```python
from build123d import *

# Parameters (mm, degrees)
SKETCH1_R           = 1
SKETCH1_R_2         = 8.1
SKETCH1_R_3         = 1.5
BOSS_EXTRUDE1_DEPTH = 3
SKETCH2_W           = 8.84
SKETCH2_H           = 1.2
CUT_EXTRUDE1_DEPTH  = 3
FILLET1_R           = 1
FILLET4_R           = 0.6


with BuildPart() as part:
    # Sketch1 → Boss-Extrude1 (new body)
    with BuildSketch(Plane(origin=(0, 0, 0), x_dir=(1, 0, 0), z_dir=(0, 1, 0))):
        Polygon((0, 0), (0, 20.3), (45, 20.3), (45, 0), (45, -3), (32.5, -3), (32.5, -13), (12.5, -13), (12.5, -3), (0, -3), align=None)
        with Locations(Location((1.4, 18.7, 0), (0, 0, 270))):
            Circle(SKETCH1_R, mode=Mode.SUBTRACT)
        with Locations(Location((1.4, 1.6, 0), (0, 0, 90))):
            Circle(SKETCH1_R, mode=Mode.SUBTRACT)
        with Locations(Location((43.6, 1.6, 0), (0, 0, 270))):
            Circle(SKETCH1_R, mode=Mode.SUBTRACT)
        with Locations(Location((43.6, 18.7, 0), (0, 0, 90))):
            Circle(SKETCH1_R, mode=Mode.SUBTRACT)
        with Locations(Location((9.58, 10.32, 0), (0, 0, 270))):
            Circle(SKETCH1_R_2, mode=Mode.SUBTRACT)
        with Locations(Location((35.42, 10.32, 0), (0, 0, 270))):
            Circle(SKETCH1_R_2, mode=Mode.SUBTRACT)
        with Locations(Location((17.5, -8, 0), (0, 0, 270))):
            Circle(SKETCH1_R_3, mode=Mode.SUBTRACT)
        with Locations(Location((27.5, -8, 0), (0, 0, 270))):
            Circle(SKETCH1_R_3, mode=Mode.SUBTRACT)
        with BuildLine():
            Line((25.675, 19.65), (19.325, 19.65))
            ThreePointArc((19.325, 19.65), (16.975, 17.3), (19.325, 14.95))
            Line((19.325, 14.95), (25.675, 14.95))
            ThreePointArc((25.675, 14.95), (28.025, 17.3), (25.675, 19.65))
        make_face(mode=Mode.SUBTRACT)
    extrude(amount=BOSS_EXTRUDE1_DEPTH)

    # Sketch2 → Cut-Extrude1 (cut)
    with BuildSketch(Plane(origin=(0, 3, 0), x_dir=(1, 0, 0), z_dir=(0, 1, 0))):
        with Locations((22.5, 1.62)):
            Rectangle(SKETCH2_W, SKETCH2_H)
    extrude(amount=-CUT_EXTRUDE1_DEPTH, mode=Mode.SUBTRACT)

    # Fillet1
    fillet1_edges = [part.edges().sort_by_distance(p)[0] for p in [
        (0, 1.5, -20.3),
        (45, 1.5, -20.3),
        (45, 1.5, 3),
        (32.5, 1.5, 3),
        (32.5, 1.5, 13),
        (12.5, 1.5, 13),
        (12.5, 1.5, 3),
        (0, 1.5, 3),
    ]]
    fillet(fillet1_edges, radius=FILLET1_R)

    # Fillet4
    fillet4_edges = [part.edges().sort_by_distance(p)[0] for p in [
        (26.92, 1.5, -2.22),
        (26.92, 1.5, -1.02),
        (18.08, 1.5, -1.02),
        (18.08, 1.5, -2.22),
    ]]
    fillet(fillet4_edges, radius=FILLET4_R - 0.0001)  # a hair under: the kernel refuses the full size


solid = part.part
```
Could you check a few things on this model? Use its own coordinates, in mm. A direction names the side the tool comes from. Round coordinates to 2 decimals unless told otherwise and drop trailing zeros. Write each loop counter-clockwise with the first axis right and the second up, starting at its lowest first coordinate (ties: lowest second). Pieces come first, ordered by that corner, then holes.
(1) If I drill on probe 1 along X at (y, z) = (1, -1.6); probe 2 along Z at (x, y) = (24, 0.45); probe 3 along X at (y, z) = (2.55, -10.5), over which ranges is the centre line in solid material (lowest first)?
Findings below:
probe 1: x = 0 to 0.4, 2.4 to 18.08, 26.92 to 42.6, 44.6 to 45
probe 2: z = -20.3 to -19.65, -14.95 to -2.22, -1.02 to 13
probe 3: x = 0 to 1.48, 17.68 to 27.32, 43.52 to 45
(2) Thinking about a two-plate mould opening in Z: for faces 1 (the face through (0.285, 1.521, 2.699)), 2 (the face through (44.44, 1.48, -1.06)), 3 (the face through (23, 0, -4)), which applies, +Z half, -Z half, draft (parallel to the pull), parting line (faces both ways), or undercut?
Findings below:
face 1: +Z half
face 2: undercut
face 3: draft
(3) Suppose I cut it at D-D on y = 1.05. State how many separate pieces and enclosed holes the cut face has, and give its area (3 significant figures).
Findings below:
separate pieces: 1
enclosed holes: 10
area: 751 mm2
(4) Suppose I cut it at C-C on z = -16. Write out the boundary of the cut face in (x, y).
Findings below:
outline: (0, 0) - (3.81, 0) - (3.81, 3) - (0, 3) - close; (15.35, 0) - (17.37, 0) - (17.37, 3) - (15.35, 3) - close; (27.63, 0) - (29.65, 0) - (29.65, 3) - (27.63, 3) - close; (41.19, 0) - (45, 0) - (45, 3) - (41.19, 3) - close
(5) Suppose I cut it at B-B on x = 35.42. Write out the boundary of the cut face in (y, z), and give its area (3 significant figures).
Findings below:
outline: (0, -20.3) - (3, -20.3) - (3, -18.42) - (0, -18.42) - close; (0, -2.22) - (3, -2.22) - (3, 3) - (0, 3) - close
area: 21.3 mm2
(6) For pin 1 (0.9 mm diameter, centred on y = 2, z = 8.5, fed in from +X), with a flat end and sliding along its axis, tell me the tip position at first contact or that it passes through.
Findings below:
pin 1: stops at x = 32.5
(7) Suppose I cut it at A-A on z = -10.32. Write out the boundary of the cut face in (x, y).
Findings below:
outline: (0, 0) - (1.48, 0) - (1.48, 3) - (0, 3) - close; (17.68, 0) - (27.32, 0) - (27.32, 3) - (17.68, 3) - close; (43.52, 0) - (45, 0) - (45, 3) - (43.52, 3) - close
(8) Which directions (+Z, -Z, +X, -X, +Y, -Y) give clear straight access to the entire face, cutting with the end or side of a thin tool? Please do faces 4 (the face through (44.699, 1.521, -20.015)), 5 (the face through (22, 1, -14.95)).
Findings below:
face 4: -Z, +X, +Y, -Y
face 5: +Y, -Y
